Part model, mm, in its own coordinate system. A direction names the side the tool comes from. Give positions to 0.01 mm unless a question says otherwise; leave off trailing zeros. Write each loop counter-clockwise with the first axis right and the second up, starting at its lowest first coordinate (ties: lowest second). Pieces come first, ordered by that corner, then holes. Notation, with made-up numbers: M 85,4 L 139,4 A33 ccw 139,36 Z; hole C 33.25,5 d5. An arc over 180 degrees is marked long. Answer as CSV lines item,"result". Start each with the question number.
Item 1: 3-axis set-ups, long thin cutter, end or side, ignore diameter. For faces 4 (the flat face through (44.6, 2.6, 6)), 5 (the flat face through (-1, 0, 1)), 6 (the flat face through (-1, 4, 10)): which of +Z, -Z, +X, -X, +Y, -Y reach the whole face in a straight line?
Item 2: Two-plate mould, pull along X, no slides. Class faces 1 (the cylindrical face through (44.3, 4.07, 8.03)), 2 (the flat face through (-1, 8, 1)), 3 (the flat face through (-75, 4, 4)): +X half, -X half, draft (parallel to the pull), parting line (faces both ways), or undercut.
Item 3: Pin check, flat tips, straight feed: pin 1 (4 mm diameter, centred on x = -46, y = 4, fed in from -Z); pin 2 (2 mm diameter, centred on x = -33, z = -7, fed in from -Y); pin 3 (4 mm diameter, centred on x = 4, y = 2, fed in from +Z); pin 4 (3 mm diameter, centred on x = 55, y = 4, fed in from +Z). Stop position of each tip, or through.
Item 4: Wall check: L1, parallel to X at y = 6.75, z = 1; L2, parallel to X at y = 2.5, z = 1.25; L3, parallel to Y at x = -46, z = 9. Give the ranges that are in metal, low to high. Write a range as from..to.
Item 5: Band-saw the part on B-B, the plane z = -8.5. List the corners of the cut face in (x, y).
Item 6: Band-saw the part on C-C, the plane x = -55. List the corners of the cut face in (y, z).
Item 7: Band-saw the part on A-A, the plane x = 46. List the corners of the cut face in (y, z), then the cut area to 3 significant figures.
Item 8: Band-saw the part on D-D, the plane x = 64. List the corners of the cut face in (y, z), then the cut area to 3 significant figures.
from build123d import *

# Parameters (mm, degrees)
EXTRUDE_1_DEPTH              = 8
HOLE_WIZARD_M3_1_D           = 3.4
HOLE_WIZARD_M3_1_CBORE_D     = 6.5
HOLE_WIZARD_M3_1_CBORE_DEPTH = 16
SKETCH_4_R                   = 2.6
CUT_EXTRUDE_1_DEPTH          = 10


with BuildPart() as part:
    # 草图1 → 凸台-拉伸1 (new body)
    with BuildSketch(Plane(origin=(0, 0, 0), x_dir=(1, 0, 0), z_dir=(0, 1, 0))):
        Polygon((-75, -10), (-49, -10), (49, -10), (75, -10), (75, 10), (-75, 10), align=None)
        with BuildLine():
            ThreePointArc((-75, -17.651517996), (-62.551252042, -11.952594339), (-49, -10))
            Line((-49, -10), (-75, -10))
            Line((-75, -10), (-75, -17.651517996))
        make_face()
        with BuildLine():
            Line((75, -10), (49, -10))
            ThreePointArc((49, -10), (62.551252042, -11.952594339), (75, -17.651517996))
            Line((75, -17.651517996), (75, -10))
        make_face()
    extrude(amount=EXTRUDE_1_DEPTH)

    # M3 六角凹头螺钉的柱形沉头孔1 (through all)
    with Locations(Plane(origin=(46, 4, -10), x_dir=(-1, 0, 0), z_dir=(0, 0, -1))):
        with Locations((0, 0), (92, 0)):
            CounterBoreHole(HOLE_WIZARD_M3_1_D / 2, HOLE_WIZARD_M3_1_CBORE_D / 2, HOLE_WIZARD_M3_1_CBORE_DEPTH)

    # 草图4 → 切除-拉伸1 (cut)
    with BuildSketch(Plane(origin=(0, 0, -10), x_dir=(-1, 0, 0), z_dir=(0, 0, -1))):
        with Locations((-55, 4)):
            Circle(SKETCH_4_R)
        with Locations((55, 4)):
            Circle(SKETCH_4_R)
    extrude(amount=-CUT_EXTRUDE_1_DEPTH, mode=Mode.SUBTRACT)


solid = part.part
Output:
1,face 4,"-Z"
1,face 5,"+Z, -Z, +X, -X, -Y"
1,face 6,"+Z, +Y, -Y"
2,face 1,"undercut"
2,face 2,"draft"
2,face 3,"-X half"
3,pin 1,"z = 6"
3,pin 2,"y = 0"
3,pin 3,"z = 10"
3,pin 4,"z = 10.59"
4,L1,"-75..-47.73, -44.27..44.27, 47.73..75"
4,L2,"-75..-48.88, -43.12..43.12, 48.88..75"
4,L3,"0..2.3, 5.7..8"
5,outline,"M -75,0 L 75,0 L 75,8 L -75,8 Z; hole C -55,4 d5.2; hole C -46,4 d6.5; hole C 46,4 d6.5; hole C 55,4 d5.2"
6,outline,"M 0,-10 L 1.4,-10 L 1.4,0 L 6.6,0 L 6.6,-10 L 8,-10 L 8,10.38 L 0,10.38 Z"
7,outline,"M 0,-10 L 0.75,-10 L 0.75,6 L 2.3,6 L 2.3,10 L 0,10 Z; M 5.7,6 L 7.25,6 L 7.25,-10 L 8,-10 L 8,10 L 5.7,10 Z"
7,area,"42.4 mm²"
8,outline,"M 0,-10 L 8,-10 L 8,12.4 L 0,12.4 Z"
8,area,"179 mm²"
